For this review, take the finished solid that the model builds, in its own axes (mm). A direction names the side the tool comes from. Give positions to 0.01 mm unless a question says otherwise; leave off trailing zeros.
1) Machinability: for faces 5 (the face through (53.15, -16.99, 0.17)), 6 (the face through (40.999, -10, 0)), which of the approach directions +Z, -Z, +X, -X, +Y, -Y give a long, thin tool a straight path to every point of the face, cutting with its end or side? Answer none if there is none.
2) Wall thickness on line 1 along Z through (x, y) = (-27.5, -10.25); line 2 along X through (y, z) = (-10.5, 3.5); line 3 along Y through (x, z) = (-25.5, 6.5): over which ranges is each line inside the solid? List them lowest first.
3) Draft analysis for pull direction Z (two halves, no side actions). For faces 1 (the face through (53.15, -3.01, 0.17)), 2 (the face through (-39.796, -10.436, 11.257)), 3 (the face through (-0.57, -3.01, 24.55)), 4 (the face through (-1, -0.6, 0)), state which applies: pulls with the +Z half, pulls with the -Z half, needs draft (parallel to the pull), parting line crosses it, or undercut.
4) For P1, Ø10, axis at x = 19.5, z = 4, coming from the -Y side; P2, Ø4, axis at x = -43.5, y = -7, coming from the -Z side; P3, Ø6, axis at x = 41.5, z = 20.5, coming from the +Y side; P4, Ø1, axis at y = -16, z = -5, coming from the +X side, all flat-tipped, find the tip position at first contact; note any pin that passes through.
from build123d import *

# Parameters (mm, degrees)
F1_DEPTH = 20
F2_R     = 9.99999
F4_DEPTH = 19.4


# Not quite as in the source:
# - a fillet or chamfer is up to 0.001 mm smaller than in the source, because OpenCascade refuses the exact size


with BuildPart() as f1:
    # F0 (on Front) → F1 (new body)
    with BuildSketch(Plane.XZ):
        with BuildLine():
            ThreePointArc((55.998519063, 12.3981075734), (51.6051207808, 23.0047092912), (40.998519063, 27.3981075734))
            Line((40.998519063, 27.3981075734), (-40.998519063, 27.3981075734))
            ThreePointArc((-40.998519063, 27.3981075734), (-51.6051207808, 23.0047092912), (-55.998519063, 12.3981075734))
            Line((-55.998519063, 12.3981075734), (-55.998519063, -12.3981075734))
            ThreePointArc((-55.998519063, -12.3981075734), (-51.6051207808, -23.0047092912), (-40.998519063, -27.3981075734))
            Line((-40.998519063, -27.3981075734), (40.998519063, -27.3981075734))
            ThreePointArc((40.998519063, -27.3981075734), (51.6051207808, -23.0047092912), (55.998519063, -12.3981075734))
            Line((55.998519063, -12.3981075734), (55.998519063, 12.3981075734))
        make_face()
    extrude(amount=F1_DEPTH)

    # F2 (radius 10 in the source; OpenCascade refuses exactly that, so slightly less here)
    f2_edges = [f1.edges().sort_by_distance(p)[0] for p in [
        (55.998519, -20, 0),
        (51.605121, -20, 23.004709),
        (0, -20, 27.398108),
        (-51.605121, -20, 23.004709),
        (-55.998519, -20, 0),
        (-51.605121, -20, -23.004709),
        (0, -20, -27.398108),
        (51.605121, -20, -23.004709),
        (0, 0, 27.398108),
    ]]
    fillet(f2_edges, radius=F2_R)

    # F3 (on face) → F4 (cut)
    with BuildSketch(Plane.XZ.offset(20)):
        with BuildLine():
            ThreePointArc((-40.998519063, -8.3981075734), (-39.8269461877, -11.2265346981), (-36.998519063, -12.3981075734))
            Line((-36.998519063, -12.3981075734), (36.998519063, -12.3981075734))
            ThreePointArc((36.998519063, -12.3981075734), (39.8269461877, -11.2265346981), (40.998519063, -8.3981075734))
            Line((40.998519063, -8.3981075734), (40.998519063, 8.3981075734))
            ThreePointArc((40.998519063, 8.3981075734), (39.8269461877, 11.2265346981), (36.998519063, 12.3981075734))
            Line((36.998519063, 12.3981075734), (-36.998519063, 12.3981075734))
            ThreePointArc((-36.998519063, 12.3981075734), (-39.8269461877, 11.2265346981), (-40.998519063, 8.3981075734))
            Line((-40.998519063, 8.3981075734), (-40.998519063, -8.3981075734))
        make_face()
    extrude(amount=-F4_DEPTH, mode=Mode.SUBTRACT)


solid = f1.part
Results list:
1. face 5: +Z, -Z, +X, -Y
1. face 6: -Y
2. line 1: z = -27.39 to -12.4, 12.4 to 27.39
2. line 2: x = -55.99 to -41, 41 to 55.99
2. line 3: y = -0.6 to 0
3. face 1: needs draft
3. face 2: undercut
3. face 3: pulls with the +Z half
3. face 4: undercut
4. P1: stops at y = -0.6
4. P2: stops at z = -27.24
4. P3: stops at y = 0
4. P4: stops at x = 54.35
